```python
from build123d import *

# Parameters (mm, degrees)
BOSS_EXTRUDE1_DEPTH = 5.08
SKETCH2_W           = 5.08
SKETCH2_H           = 15.24
SKETCH2_H_2         = 10.16
SKETCH2_H_3         = 5.08
SKETCH2_W_2         = 7.62
SKETCH2_W_3         = 12.7
CUT_EXTRUDE1_DEPTH  = 5.08


with BuildPart() as part:
    # Sketch1 → Boss-Extrude1 (new body)
    with BuildSketch(Plane.XY):
        Polygon((0, 0), (0, 76.2), (5.08, 76.2), (38.1, 5.08), (38.1, 0), align=None)
    extrude(amount=BOSS_EXTRUDE1_DEPTH)

    # Sketch2 → Cut-Extrude1 (cut)
    with BuildSketch(Plane.XY.offset(5.08)):
        with Locations((2.54, 68.58)):
            Rectangle(SKETCH2_W, SKETCH2_H)
        with Locations((2.54, 38.1)):
            Rectangle(SKETCH2_W, SKETCH2_H)
        with Locations((2.54, 10.16)):
            Rectangle(SKETCH2_W, SKETCH2_H_2)
        with Locations((2.54, 2.54)):
            Rectangle(SKETCH2_W, SKETCH2_H_3)
        with Locations((8.89, 2.54)):
            Rectangle(SKETCH2_W_2, SKETCH2_H_3)
        with Locations((31.75, 2.54)):
            Rectangle(SKETCH2_W_3, SKETCH2_H_3)
    extrude(amount=-CUT_EXTRUDE1_DEPTH, mode=Mode.SUBTRACT)


solid = part.part
```
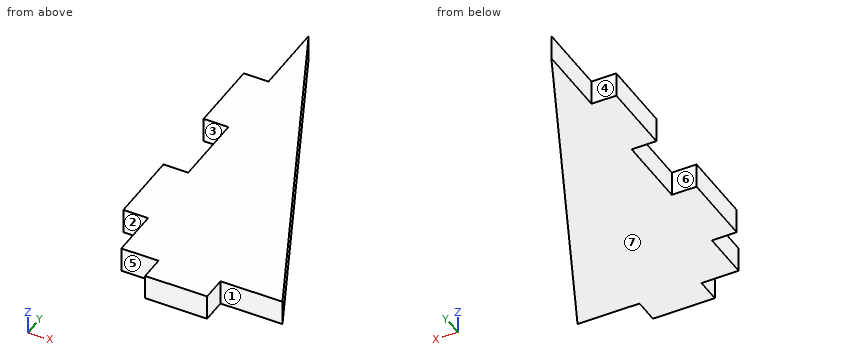
Design review of the part built by this model. Coordinates are the model's own, in mm. Face numbers are marked on the shaded views. A direction names the side the tool comes from. Coordinates: 2 decimals unless noted, no trailing zeros. Write each loop counter-clockwise with the first axis right and the second up, starting at its lowest first coordinate (ties: lowest second). Pieces come first, ordered by that corner, then holes.
1) Add section B-B (x = 30). Write out the cut boundary in (y, z), plus the area to 3 significant figures.
2) Add section C-C (y = 59). Write out the cut boundary in (x, z).
3) Insertion check: pin 1 (2.5 mm diameter, centred on y = 2, z = 2.5, fed in from -X); pin 2 (1 mm diameter, centred on x = 29, z = 4.5, fed in from +Y); pin 3 (2 mm diameter, centred on y = 42, z = 4, fed in from -X). Each pin has a flat end and moves straight along its axis. Give the tip position at first contact, or say it passes through.
4) Machinability: for the marked faces 1, 2 and 3, which of the approach directions +Z, -Z, +X, -X, +Y, -Y give a long, thin tool a straight path to every point of the face, cutting with its end or side? Answer none if there is none.
5) To check wall thickness, follow L1, parallel to Y at x = 2.5, z = 3.7; L2, parallel to X at y = 26, z = 4.65; L3, parallel to X at y = 45, z = 0.35. State the ranges of each line that lie inside material, in increasing order.
6) Add section A-A (z = 4.25). Write out the cut boundary in (x, y), plus the area to 3 significant figures.
7) Mouldability with a two-part tool opening along Y and no side actions: class the marked faces 4, 5, 6 and 7 as +Y half, -Y half, draft (parallel to the pull), parting line (faces both ways), or undercut.
Check result:
1. outline: (5.08, 0) - (22.53, 0) - (22.53, 5.08) - (5.08, 5.08) - close
1. area: 88.6 mm2
2. outline: (0, 0) - (13.07, 0) - (13.07, 5.08) - (0, 5.08) - close
3. pin 1: stops at x = 12.7
3. pin 2: stops at y = 25.76
3. pin 3: stops at x = 5.08
4. face 1: +Z, -Z, +X, -Y
4. face 2: +Z, -Z, -X, -Y
4. face 3: +Z, -Z, -X
5. L1: y = 15.24 to 30.48, 45.72 to 60.96
5. L2: x = 0 to 28.39
5. L3: x = 5.08 to 19.57
6. outline: (0, 15.24) - (5.08, 15.24) - (5.08, 5.08) - (12.7, 5.08) - (12.7, 0) - (25.4, 0) - (25.4, 5.08) - (38.1, 5.08) - (5.08, 76.2) - (5.08, 60.96) - (0, 60.96) - (0, 45.72) - (5.08, 45.72) - (5.08, 30.48) - (0, 30.48) - close
6. area: 1,390 mm2
7. face 4: +Y half
7. face 5: -Y half
7. face 6: undercut
7. face 7: draft
